from build123d import *

# Parameters (mm, degrees)
F0_R          = 1.5
F1_DEPTH      = 16
F2_R          = 0.5
F3_DEPTH      = 2
F4_R          = 0.5
F5_DEPTH      = 2
F6_R          = 3
F6_R_2        = 1
F7_DEPTH      = 2
F7_DEPTH_BACK = 2
F8_R          = 1
F9_DEPTH      = 2
F9_DEPTH_BACK = 2


with BuildPart() as f1:
    # F0 (on Top) → F1 (new body)
    with BuildSketch(Plane.XY):
        Circle(F0_R)
    extrude(amount=F1_DEPTH)

    # F2 (on face) → F3 (cut)
    with BuildSketch(Plane.XY.offset(16)):
        Circle(F2_R)
    extrude(amount=-F3_DEPTH, mode=Mode.SUBTRACT)

    # F4 (on face) → F5 (cut)
    with BuildSketch(Plane(origin=(0, 0, 0), x_dir=(1, 0, 0), z_dir=(0, 0, -1))):
        Circle(F4_R)
    extrude(amount=-F5_DEPTH, mode=Mode.SUBTRACT)

    # F6 (on Front) → F7 (join, two sides)
    with BuildSketch(Plane.XZ) as f7_sk:
        with Locations((0, 8)):
            Circle(F6_R)
        with Locations((0, 8)):
            Circle(F6_R_2, mode=Mode.SUBTRACT)
    extrude(amount=F7_DEPTH)
    extrude(f7_sk.sketch, amount=-F7_DEPTH_BACK)

    # F8 (on Front) → F9 (cut, two sides)
    with BuildSketch(Plane.XZ) as f9_sk:
        with Locations((0, 8)):
            Circle(F8_R)
    extrude(amount=-F9_DEPTH, mode=Mode.SUBTRACT)
    extrude(f9_sk.sketch, amount=F9_DEPTH_BACK, mode=Mode.SUBTRACT)


solid = f1.part
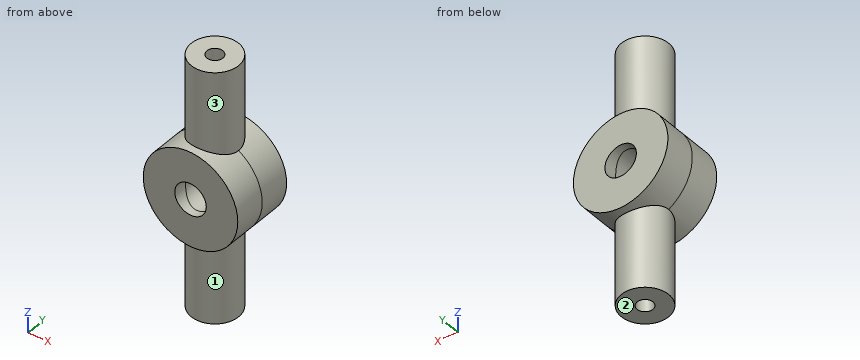
Read the model definition and answer for the solid it produces. Units are mm, in the model's axes. Face numbers are marked on the shaded views. A direction names the side the tool comes from. Round coordinates to 2 decimals unless told otherwise and drop trailing zeros. Loops run counter-clockwise (first coordinate to the right, second up) from the corner with the lowest first, then second, coordinate; pieces in that order, holes last.
Q1. Each of these flat-tipped pins is pushed along its axis until it touches: pin 1 (0.8 mm diameter, centred on x = 0, y = 0, fed in from +Z); pin 2 (3 mm diameter, centred on x = 0, z = 8, fed in from +Y); pin 3 (1.6 mm diameter, centred on x = 0, z = 8, fed in from +Y); pin 4 (3 mm diameter, centred on x = -0.5, z = 2.5, fed in from -Y). Where does it stop, or does it pass through?
Q2. Section B-B on z = 8 is taken. Write down the section's boundary in (x, y), and give its area (3 significant figures).
Q3. Section C-C on y = 0.65 is taken. Write down the section's boundary in (x, z), and give its area (3 significant figures).
Q4. Which of the six approach directions +Z, -Z, +X, -X, +Y, -Y give full straight-line access (tool end or side, diameter ignored) to the marked faces 1, 2 and 3?
Q5. Section A-A on x = 0 is taken. Write down the section's boundary in (y, z).
Q6. Consider probe 1 along Z at (x, y) = (0, -1.25); probe 2 along Z at (x, y) = (0, 1.7); probe 3 along Z at (x, y) = (1.5, 1.3). Determine where each line is inside the solid, lowest interval first.
Q7. Section D-D on x = 1.25 is taken. Write down the section's boundary in (y, z), and give its area (3 significant figures).
Output:
1. pin 1: stops at z = 14
1. pin 2: stops at y = 2
1. pin 3: passes through
1. pin 4: stops at y = -1.5
2. outline: (-3, -2) - (-1, -2) - (-1, 2) - (-3, 2) - close; (1, -2) - (3, -2) - (3, 2) - (1, 2) - close
2. area: 16.0 mm2
3. outline: (-1.35, 0) - (1.35, 0) - (1.35, 5.32) arc R3 ccw to (1.35, 10.68) - (1.35, 16) - (-1.35, 16) - (-1.35, 10.68) arc R3 ccw to (-1.35, 5.32) - close; hole circle Ø2 at (0, 8)
3. area: 52.7 mm2
4. face 1: -Z
4. face 2: -Z, +X, -X, +Y, -Y
4. face 3: +Z
5. outline: (-2, 5) - (-1.5, 5) - (-1.5, 0) - (-0.5, 0) - (-0.5, 2) - (0.5, 2) - (0.5, 0) - (1.5, 0) - (1.5, 5) - (2, 5) - (2, 7) - (-2, 7) - close; (-2, 9) - (2, 9) - (2, 11) - (1.5, 11) - (1.5, 16) - (0.5, 16) - (0.5, 14) - (-0.5, 14) - (-0.5, 16) - (-1.5, 16) - (-1.5, 11) - (-2, 11) - close
6. probe 1: z = 0 to 7, 9 to 16
6. probe 2: z = 5 to 7, 9 to 11
6. probe 3: z = 5.4 to 10.6
7. outline: (-2, 5.27) - (-0.83, 5.27) - (-0.83, 0) - (0.83, 0) - (0.83, 5.27) - (2, 5.27) - (2, 10.73) - (0.83, 10.73) - (0.83, 16) - (-0.83, 16) - (-0.83, 10.73) - (-2, 10.73) - close
7. area: 39.3 mm2
